CAD build for the part. Positions are in the model's coordinates, mm. Face numbers are marked on the shaded views. Coordinates: 2 decimals unless noted, no trailing zeros. Write each loop counter-clockwise with the first axis right and the second up, starting at its lowest first coordinate (ties: lowest second). Pieces come first, ordered by that corner, then holes. Notation, with made-up numbers: (24.25, 35.25) -> (49.25, 35.25) arc R18 cw to (49.25, 42.25) -> close; hole circle Ø4 at (86, -5). An arc over 180 degrees is marked (long way). Answer as CSV lines item,"result".
```python
from build123d import *
from build123d.topology import SkipClean

# Parameters (mm, degrees)
CROQUIS1_R                   = 95
SALIENTE_EXTRUIR1_DEPTH      = 106
CROQUIS2_R                   = 83
CORTAR_EXTRUIR1_DEPTH        = 100
CROQUIS3_R                   = 90.5
CORTAR_EXTRUIR2_DEPTH        = 12
CROQUIS4_R                   = 17
CORTAR_EXTRUIR4_DEPTH        = 89
SALIENTE_EXTRUIR2_DEPTH      = 0.001
SALIENTE_EXTRUIR2_DEPTH_BACK = 89
CROQUIS5_R                   = 3.925
CORTAR_EXTRUIR5_DEPTH        = 79
CORTAR_EXTRUIR5_DEPTH_BACK   = 79
CROQUIS6_R                   = 3.925
CORTAR_EXTRUIR6_START        = 81.240384105
CORTAR_EXTRUIR6_DEPTH        = 7.759615895
CROQUIS7_R                   = 3.925
SALIENTE_EXTRUIR3_DEPTH      = 10
CORTAR_EXTRUIR10_START       = 81.240383801
CORTAR_EXTRUIR10_DEPTH       = 7.759616199
CROQUIS8_R                   = 3.925
SALIENTE_EXTRUIR4_DEPTH      = 10
REDONDEO2_R                  = 2
CORTAR_EXTRUIR11_DEPTH       = 21
CROQUIS13_R                  = 2.5
CORTAR_EXTRUIR12_DEPTH       = 10
CROQUIS14_R                  = 95
CORTAR_EXTRUIR13_DEPTH       = 60
CROQUIS15_R                  = 95
SALIENTE_EXTRUIR5_DEPTH      = 2.5
CORTAR_EXTRUIR14_DEPTH       = 5
CROQUIS17_R                  = 4
CORTAR_EXTRUIR16_DEPTH       = 5


# Read off the part's stored shape, not the designer's step: Cortar-Extruir6, Cortar-Extruir10
with BuildPart() as part:
    # Croquis1 → Saliente-Extruir1 (new body)
    with BuildSketch(Plane.XY):
        Circle(CROQUIS1_R)
    extrude(amount=SALIENTE_EXTRUIR1_DEPTH)

    # Croquis2 → Cortar-Extruir1 (cut)
    with BuildSketch(Plane.XY.offset(106)):
        Circle(CROQUIS2_R)
    extrude(amount=-CORTAR_EXTRUIR1_DEPTH, mode=Mode.SUBTRACT)

    # Croquis3 → Cortar-Extruir2 (cut)
    with BuildSketch(Plane.XY.offset(106)):
        Circle(CROQUIS3_R)
    extrude(amount=-CORTAR_EXTRUIR2_DEPTH, mode=Mode.SUBTRACT)

    # Croquis4 → Cortar-Extruir4 (cut)
    with BuildSketch(Plane(origin=(0, 0, 0), x_dir=(0, 0, -1), z_dir=(1, 0, 0))):
        with Locations((-83, 0)):
            Circle(CROQUIS4_R)
    extrude(amount=-CORTAR_EXTRUIR4_DEPTH, mode=Mode.SUBTRACT)

    # Croquis5 → Saliente-Extruir2 (add, two sides: drawn at the far end of the back side and taken through both)
    with BuildSketch(Plane(origin=(0, 0, 0), x_dir=(0, 0, -1), z_dir=(1, 0, 0)).offset(-SALIENTE_EXTRUIR2_DEPTH_BACK)):
        with Locations((-85, 0)):
            Circle(CROQUIS5_R)
    extrude(amount=SALIENTE_EXTRUIR2_DEPTH + SALIENTE_EXTRUIR2_DEPTH_BACK)

    # Croquis6 → Cortar-Extruir5 (cut, two sides: drawn at the far end of the back side and taken through both)
    with BuildSketch(Plane(origin=(0, 0, 0), x_dir=(0, 0, -1), z_dir=(1, 0, 0)).offset(-CORTAR_EXTRUIR5_DEPTH_BACK)):
        with Locations((-85, 0)):
            Circle(CROQUIS6_R)
    extrude(amount=CORTAR_EXTRUIR5_DEPTH + CORTAR_EXTRUIR5_DEPTH_BACK, mode=Mode.SUBTRACT)

    # Cortar-Extruir6 outline → Cortar-Extruir6 (cut)
    with BuildSketch(Plane(origin=(0, 0, 0), x_dir=(0.8191520442889906, 0.5735764363510478, 0), z_dir=(0.5735764363510478, -0.8191520442889907, 0)).offset(CORTAR_EXTRUIR6_START)):
        with BuildLine():
            Line((12.961481397, 94), (-12.961481397, 94))
            ThreePointArc((-12.961481397, 94), (0, 66), (12.961481397, 94))
        make_face()
    extrude(amount=CORTAR_EXTRUIR6_DEPTH, mode=Mode.SUBTRACT)

    # Croquis7 → Saliente-Extruir3 (add)
    with BuildSketch(Plane(origin=(51.048302836, -72.904531941, 0), x_dir=(0.8191520442843079, 0.5735764363577354, 2.1722123141071213e-13), z_dir=(-0.5735764363577354, 0.8191520442843079, 3.1022406865588427e-13))):
        with Locations((0, -85)):
            Circle(CROQUIS7_R)
    extrude(amount=SALIENTE_EXTRUIR3_DEPTH)

    # Cortar-Extruir10 outline → Cortar-Extruir10 (cut)
    with BuildSketch(Plane(origin=(0, 0, 0), x_dir=(0.7660444431189818, -0.642787609686535, 0), z_dir=(0.6427876096865349, 0.7660444431189818, 0)).offset(CORTAR_EXTRUIR10_START)):
        with BuildLine():
            Line((-14.422205102, -94), (14.422205102, -94))
            ThreePointArc((14.422205102, -94), (0, -68), (-14.422205102, -94))
        make_face()
    extrude(amount=CORTAR_EXTRUIR10_DEPTH, mode=Mode.SUBTRACT)

    # Croquis8 → Saliente-Extruir4 (add)
    with BuildSketch(Plane(origin=(57.208097263, 68.177955437, 0), x_dir=(0.7660444431126934, -0.642787609694029, -3.1196544125319357e-13), z_dir=(-0.642787609694029, -0.7660444431126934, -3.717859353713491e-13))):
        with Locations(Location((0, 85, 0), (0, 0, 180))):
            Circle(CROQUIS8_R)
    extrude(amount=SALIENTE_EXTRUIR4_DEPTH)

    # Redondeo2
    redondeo2_edges = [part.edges().sort_by_distance(p)[0] for p in [
        (-89, 0, 88.925),
        (47.833131062, -75.155819454, 85),
        (60.214821702, 65.655014069, 85),
    ]]
    fillet(redondeo2_edges, radius=REDONDEO2_R)

    # Croquis12 → Cortar-Extruir11 (cut)
    with BuildSketch(Plane.XY.offset(6)):
        Polygon((-2, 6), (2, 6), (2, 2), (6, 2), (6, -2), (2, -2), (2, -6), (-2, -6), (-2, -2), (-6, -2), (-6, 2), (-2, 2), align=None)
    extrude(amount=-CORTAR_EXTRUIR11_DEPTH, mode=Mode.SUBTRACT)

    # Croquis13 → Cortar-Extruir12 (cut)
    with BuildSketch(Plane.XY.offset(6)):
        with Locations((0, 77.833820013)):
            Circle(CROQUIS13_R)
        with Locations((77.833820013, 0)):
            Circle(CROQUIS13_R)
        with Locations((0, -77.833820013)):
            Circle(CROQUIS13_R)
        with Locations((-77.833820013, 0)):
            Circle(CROQUIS13_R)
    extrude(amount=-CORTAR_EXTRUIR12_DEPTH, mode=Mode.SUBTRACT)

    # Croquis14 → Cortar-Extruir13 (cut)
    with BuildSketch(Plane(origin=(0, 0, 0), x_dir=(-1, 0, 0), z_dir=(0, 0, -1))):
        Circle(CROQUIS14_R)
    extrude(amount=-CORTAR_EXTRUIR13_DEPTH, mode=Mode.SUBTRACT)

    # Croquis15 → Saliente-Extruir5 (add, symmetric)
    with SkipClean():  # the faces are left unmerged after this step: merging them gives an invalid solid
        with BuildSketch(Plane(origin=(0, 0, 60), x_dir=(-1, 0, 0), z_dir=(0, 0, -1))):
            Circle(CROQUIS15_R)
        extrude(amount=SALIENTE_EXTRUIR5_DEPTH, both=True)
    add(part.part.scale(1), mode=Mode.REPLACE)  # the faces are merged on a copy

    # Croquis16 → Cortar-Extruir14 (cut)
    with BuildSketch(Plane(origin=(0, 0, 57.5), x_dir=(-1, 0, 0), z_dir=(0, 0, -1))):
        Polygon((-2, 6), (2, 6), (2, 2), (6, 2), (6, -2), (2, -2), (2, -6), (-2, -6), (-2, -2), (-6, -2), (-6, 2), (-2, 2), align=None)
    extrude(amount=-CORTAR_EXTRUIR14_DEPTH, mode=Mode.SUBTRACT)

    # Croquis17 → Cortar-Extruir16 (cut)
    with BuildSketch(Plane(origin=(0, 0, 57.5), x_dir=(-1, 0, 0), z_dir=(0, 0, -1))):
        with Locations((0, 73.859779167)):
            Circle(CROQUIS17_R)
        with Locations((63.964445077, 36.929889584)):
            Circle(CROQUIS17_R)
        with Locations((63.964445077, -36.929889584)):
            Circle(CROQUIS17_R)
        with Locations((0, -73.859779167)):
            Circle(CROQUIS17_R)
        with Locations((-63.964445077, -36.929889584)):
            Circle(CROQUIS17_R)
        with Locations((-63.964445077, 36.929889584)):
            Circle(CROQUIS17_R)
    extrude(amount=-CORTAR_EXTRUIR16_DEPTH, mode=Mode.SUBTRACT)


solid = part.part
```
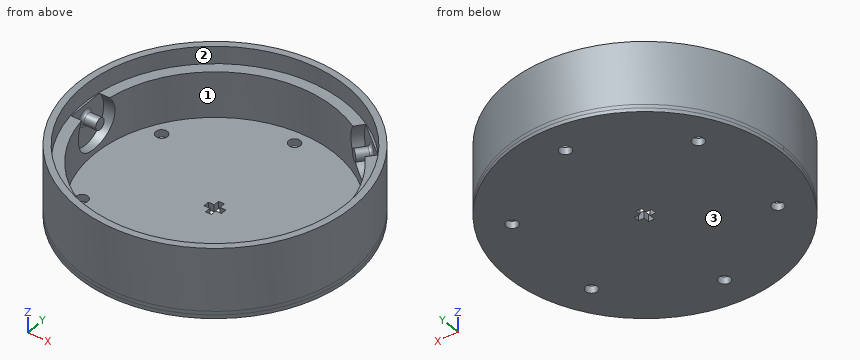
Item 1: Flat gauge pins, fed straight in: pin 1 (12 mm diameter, centred on x = 70, z = 97.5, fed in from +Y); pin 2 (1.5 mm diameter, centred on x = -49.5, y = 6, fed in from +Z); pin 3 (9 mm diameter, centred on x = 63.96, y = 36.93, fed in from -Z); pin 4 (5 mm diameter, centred on y = 68, z = 67.5, fed in from -X). Where does each tip first touch, or does it go through?
Answer below:
pin 1,"stops at y = 70.21"
pin 2,"stops at z = 62.5"
pin 3,"stops at z = 57.5"
pin 4,"stops at x = -68.81"
Item 2: Saw through at B-B on x = -18. Give the cut face in (y, z), and give its area (3 significant figures).
Answer below:
outline,"(-93.28, 57.5) -> (93.28, 57.5) -> (93.28, 106) -> (88.69, 106) -> (88.69, 94) -> (81.02, 94) -> (81.02, 62.5) -> (-81.02, 62.5) -> (-81.02, 94) -> (-88.69, 94) -> (-88.69, 106) -> (-93.28, 106) -> close"
area,"1,810 mm2"
Item 3: Saw through at C-C on y = 22. Give the cut face in (x, z), and give its area (3 significant figures).
Answer below:
outline,"(-92.42, 57.5) -> (92.42, 57.5) -> (92.42, 106) -> (87.79, 106) -> (87.79, 94) -> (80.03, 94) -> (80.03, 62.5) -> (-80.03, 62.5) -> (-80.03, 94) -> (-87.79, 94) -> (-87.79, 106) -> (-92.42, 106) -> close"
area,"1,820 mm2"
Item 4: Wall check: line 1 (X direction, y = 60, z = 85.5); line 2 (X direction, y = -2, z = 66); line 3 (X direction, y = 0, z = 83.5). Give the ranges that are in metal, low to high. Write a range as from..to.
Answer below:
line 1,"x = -73.65..-57.35, 51.4..55.43, 66.95..73.65"
line 2,"x = -94.98..-82.98, 82.98..94.98"
line 3,"x = -95..-79, 83..95"
Item 5: Saw through at D-D on z = 98.5. Give the cut face in (x, y), and give its area (3 significant figures).
Answer below:
outline,"circle Ø190 at (0, 0); hole circle Ø181 at (0, 0)"
area,"2,620 mm2"
Item 6: Saw through at A-A on z = 72. Give the cut face in (x, y), and give its area (3 significant figures).
Answer below:
outline,"circle Ø190 at (0, 0); hole (-89, -12.96) -> (-81.98, -12.96) arc R83 ccw to (36.41, -74.59) -> (40.43, -80.34) -> (61.67, -65.47) -> (57.64, -59.72) arc R83 ccw to (61.28, 55.98) -> (65.6, 61.14) -> (48.82, 75.22) -> (44.49, 70.07) arc R83 ccw to (-81.98, 12.96) -> (-89, 12.96) -> close"
area,"6,250 mm2"
Item 7: Two-plate mould, pull along X, no slides. Class the marked faces 1, 2 and 3: pulls with the +X half, pulls with the -X half, needs draft (parallel to the pull), parting line crosses it, or undercut.
Answer below:
face 1,"undercut"
face 2,"undercut"
face 3,"needs draft"
